Answer from the drawing. Dimensions are ordinates in mm from the lowest x, y and z of the part. A direction names the side the tool comes from. Give positions to 0.01 mm unless a question says otherwise; leave off trailing zeros. Write each loop counter-clockwise with the first axis right and the second up, starting at its lowest first coordinate (ties: lowest second). Pieces come first, ordered by that corner, then holes.
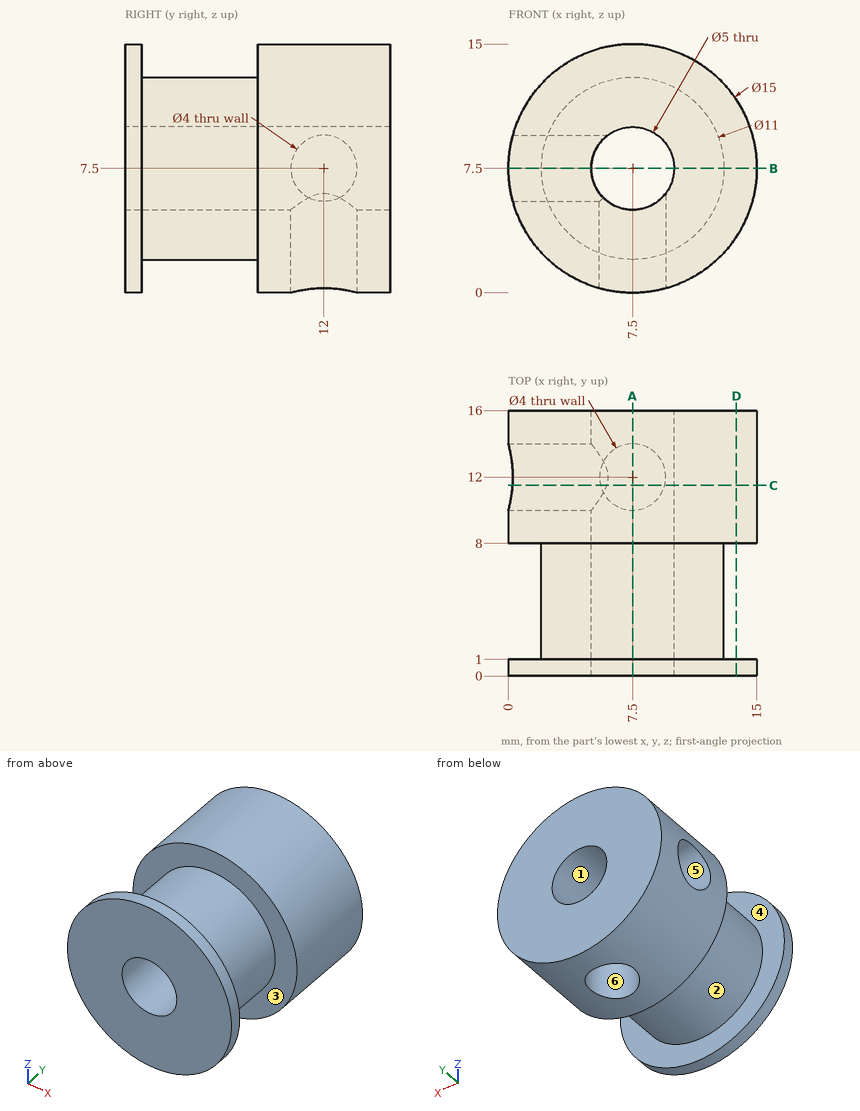
Item 1: Each of these flat-tipped pins is pushed along its axis until it touches: pin 1 Ø1.5 at (y, z) = (12, 12) entering from +X; pin 2 Ø3.5 at (x, y) = (7.5, 12) entering from -Z; pin 3 Ø2.5 at (y, z) = (12, 7.5) entering from -X. Where does it stop, or does it pass through?
Result set:
pin 1: stops at x = 14
pin 2: stops at z = 9.29
pin 3: stops at x = 9.67
Item 2: Section B-B (z = 7.5) is taken. Write down the section's boundary in (x, y), and give its area (3 significant figures).
Result set:
outline: (0, 0) - (5, 0) - (5, 10) - (0, 10) - (0, 8) - (2, 8) - (2, 1) - (0, 1) - close; (0, 14) - (5, 14) - (5, 16) - (0, 16) - close; (10, 0) - (15, 0) - (15, 1) - (13, 1) - (13, 8) - (15, 8) - (15, 16) - (10, 16) - close
area: 112 mm2
Item 3: Section A-A (x = 7.5) is taken. Write down the section's boundary in (y, z).
Result set:
outline: (0, 0) - (1, 0) - (1, 2) - (8, 2) - (8, 0) - (10, 0) - (10, 5) - (0, 5) - close; (0, 10) - (16, 10) - (16, 15) - (8, 15) - (8, 13) - (1, 13) - (1, 15) - (0, 15) - close; (14, 0) - (16, 0) - (16, 5) - (14, 5) - close
Item 4: Which of the six approach directions +Z, -Z, +X, -X, +Y, -Y give full straight-line access (tool end or side, diameter ignored) to the marked faces 4, 5 and 6?
Result set:
face 4: none
face 5: -X
face 6: -Z
Item 5: Section C-C (y = 11.5) is taken. Write down the section's boundary in (x, z), and give its area (3 significant figures).
Result set:
outline: (0.25, 5.56) arc R7.5 ccw to (5.56, 0.25) - (5.56, 5.56) - close; (0.25, 9.44) - (5.92, 9.44) arc R2.5 cw to (9.44, 5.92) - (9.44, 0.25) arc R7.5 ccw (long way) to start
area: 117 mm2
Item 6: Find the intervals of material crossed by line 1 along Y through (x, z) = (13.25, 2.75); line 2 along Y through (x, z) = (6, 3.5); line 3 along X through (y, z) = (5, 7.5), in increasing order.
Result set:
line 1: y = 0 to 1, 8 to 16
line 2: y = 0 to 10.68, 13.32 to 16
line 3: x = 2 to 5, 10 to 13
Item 7: Section D-D (x = 13.75) is taken. Write down the section's boundary in (y, z), and give its area (3 significant figures).
Result set:
outline: (0, 3.35) - (1, 3.35) - (1, 11.65) - (0, 11.65) - close; (8, 3.35) - (16, 3.35) - (16, 11.65) - (8, 11.65) - close
area: 74.6 mm2
Item 8: Determine the mould class of the marked faces 1, 2 and 3 for opening direction X: pulls with the +X half, pulls with the -X half, needs draft (parallel to the pull), parting line crosses it, or undercut.
Result set:
face 1: undercut
face 2: parting line crosses it
face 3: needs draft
